```python
from build123d import *

# Parameters (mm, degrees)
SKETCH1_R      = 26.5
SKETCH1_R_2    = 5
EXTRUDE1_DEPTH = 60
SKETCH3_R      = 2
EXTRUDE2_DEPTH = 10
EXTRUDE3_START = -41
EXTRUDE3_DEPTH = 41
EXTRUDE4_DEPTH = 19
FILLET1_R      = 1


with BuildPart() as part:
    # Sketch1 → Extrude1 (new body)
    with BuildSketch(Plane(origin=(0, 0, 0), x_dir=(0, 0, -1), z_dir=(1, 0, 0))):
        Circle(SKETCH1_R)
        Circle(SKETCH1_R_2, mode=Mode.SUBTRACT)
    extrude(amount=EXTRUDE1_DEPTH)

    # Sketch2 → Cut-Revolve1 (revolve, cut)
    with BuildSketch(Plane.XY):
        Polygon((60, 16), (60, 26.5), (41, 26.5), (41, 12), (48, 12), (48, 19), (51, 19), (51, 17.5), (57, 17.5), (57, 16), align=None)
    revolve(axis=Axis((0, 0, 0), (1, 0, 0)), mode=Mode.SUBTRACT)

    # Sketch3 → Extrude2 (cut)
    with BuildSketch(Plane(origin=(60, 0, 0), x_dir=(0, 0, -1), z_dir=(1, 0, 0))):
        with Locations((0, 12.5)):
            Circle(SKETCH3_R)
        with Locations((12.5, 0)):
            Circle(SKETCH3_R)
        with Locations((0, -12.5)):
            Circle(SKETCH3_R)
        with Locations((-12.5, 0)):
            Circle(SKETCH3_R)
    extrude(amount=-EXTRUDE2_DEPTH, mode=Mode.SUBTRACT)

    # Sketch4 → Extrude3 (cut)
    with BuildSketch(Plane.ZY.offset(EXTRUDE3_START)):
        with BuildLine():
            Line((0, 14.5), (1.048050077, 26.479267192))
            ThreePointArc((1.048050077, 26.479267192), (0, 26.5), (-1.048050077, 26.479267192))
            Line((-1.048050077, 26.479267192), (0, 14.5))
        make_face()
        with BuildLine():
            Line((11.377526787, 23.933279846), (6.738485995, 12.839112372))
            Line((6.738485995, 12.839112372), (13.233531299, 22.959173534))
            ThreePointArc((13.233531299, 22.959173534), (12.315164059, 23.46458468), (11.377526787, 23.933279846))
        make_face()
        with BuildLine():
            Line((-6.738485995, 12.839112372), (-11.377526787, 23.933279846))
            ThreePointArc((-11.377526787, 23.933279846), (-12.315164059, 23.46458468), (-13.233531299, 22.959173534))
            Line((-13.233531299, 22.959173534), (-6.738485995, 12.839112372))
        make_face()
        with BuildLine():
            Line((21.196649379, 15.904466515), (11.933266055, 8.236938828))
            Line((11.933266055, 8.236938828), (22.387369981, 14.179409907))
            ThreePointArc((22.387369981, 14.179409907), (21.809072446, 15.053715788), (21.196649379, 15.904466515))
        make_face()
        with BuildLine():
            Line((-11.933266055, 8.236938828), (-21.196649379, 15.904466515))
            ThreePointArc((-21.196649379, 15.904466515), (-21.809072446, 15.053715788), (-22.387369981, 14.179409907))
            Line((-22.387369981, 14.179409907), (-11.933266055, 8.236938828))
        make_face()
        with BuildLine():
            Line((26.159875044, 4.232131575), (14.394278674, 1.747781864))
            Line((14.394278674, 1.747781864), (26.412531998, 2.151314351))
            ThreePointArc((26.412531998, 2.151314351), (26.306785164, 3.194222027), (26.159875044, 4.232131575))
        make_face()
        with BuildLine():
            Line((-14.394278674, 1.747781864), (-26.159875044, 4.232131575))
            ThreePointArc((-26.159875044, 4.232131575), (-26.306785164, 3.194222027), (-26.412531998, 2.151314351))
            Line((-26.412531998, 2.151314351), (-14.394278674, 1.747781864))
        make_face()
        with BuildLine():
            Line((25.130188598, -8.409733707), (13.557735519, -5.141770862))
            Line((13.557735519, -5.141770862), (24.38690124, -10.369621396))
            ThreePointArc((24.38690124, -10.369621396), (24.777930431, -9.397029507), (25.130188598, -8.409733707))
        make_face()
        with BuildLine():
            Line((-13.557735519, -5.141770862), (-25.130188598, -8.409733707))
            ThreePointArc((-25.130188598, -8.409733707), (-24.777930431, -9.397029507), (-24.38690124, -10.369621396))
            Line((-24.38690124, -10.369621396), (-13.557735519, -5.141770862))
        make_face()
        with BuildLine():
            Line((18.343478796, -19.125030344), (9.615278544, -10.853405848))
            Line((9.615278544, -10.853405848), (16.774525302, -20.51500185))
            ThreePointArc((16.774525302, -20.51500185), (17.572750443, -19.835534827), (18.343478796, -19.125030344))
        make_face()
        with BuildLine():
            Line((-9.615278544, -10.853405848), (-18.343478796, -19.125030344))
            ThreePointArc((-18.343478796, -19.125030344), (-17.572750443, -19.835534827), (-16.774525302, -20.51500185))
            Line((-16.774525302, -20.51500185), (-9.615278544, -10.853405848))
        make_face()
        with BuildLine():
            Line((7.354499064, -25.459013011), (3.470077132, -14.078656353))
            Line((3.470077132, -14.078656353), (5.319307772, -25.960642612))
            ThreePointArc((5.319307772, -25.960642612), (6.341865104, -25.729958162), (7.354499064, -25.459013011))
        make_face()
        with BuildLine():
            Line((-3.470077132, -14.078656353), (-7.354499064, -25.459013011))
            ThreePointArc((-7.354499064, -25.459013011), (-6.341865104, -25.729958162), (-5.319307772, -25.960642612))
            Line((-5.319307772, -25.960642612), (-3.470077132, -14.078656353))
        make_face()
    extrude(amount=EXTRUDE3_DEPTH, mode=Mode.SUBTRACT)

    # Sketch5 → Extrude4 (cut)
    with BuildSketch(Plane(origin=(60, 0, 0), x_dir=(0, 0, -1), z_dir=(1, 0, 0))):
        with BuildLine():
            Line((-5, 9.346657156), (-5, 15.198684154))
            ThreePointArc((-5, 15.198684154), (-11.313708499, 11.313708499), (-15.198684154, 5))
            Line((-15.198684154, 5), (-9.346657156, 5))
            ThreePointArc((-9.346657156, 5), (-7.495331881, 7.495331881), (-5, 9.346657156))
        make_face()
        with BuildLine():
            Line((-5, 15.198684154), (-5, 18.33030278))
            ThreePointArc((-5, 18.33030278), (-13.435028843, 13.435028843), (-18.33030278, 5))
            Line((-18.33030278, 5), (-15.198684154, 5))
            ThreePointArc((-15.198684154, 5), (-11.313708499, 11.313708499), (-5, 15.198684154))
        make_face()
        with BuildLine():
            ThreePointArc((15.198684154, 5), (11.313708499, 11.313708499), (5, 15.198684154))
            Line((5, 15.198684154), (5, 9.346657156))
            ThreePointArc((5, 9.346657156), (7.495331881, 7.495331881), (9.346657156, 5))
            Line((9.346657156, 5), (15.198684154, 5))
        make_face()
        with BuildLine():
            ThreePointArc((18.33030278, 5), (13.435028843, 13.435028843), (5, 18.33030278))
            Line((5, 18.33030278), (5, 15.198684154))
            ThreePointArc((5, 15.198684154), (11.313708499, 11.313708499), (15.198684154, 5))
            Line((15.198684154, 5), (18.33030278, 5))
        make_face()
        with BuildLine():
            ThreePointArc((5, -15.198684154), (11.313708499, -11.313708499), (15.198684154, -5))
            Line((15.198684154, -5), (9.346657156, -5))
            ThreePointArc((9.346657156, -5), (7.495331881, -7.495331881), (5, -9.346657156))
            Line((5, -9.346657156), (5, -15.198684154))
        make_face()
        with BuildLine():
            ThreePointArc((5, -18.33030278), (13.435028843, -13.435028843), (18.33030278, -5))
            Line((18.33030278, -5), (15.198684154, -5))
            ThreePointArc((15.198684154, -5), (11.313708499, -11.313708499), (5, -15.198684154))
            Line((5, -15.198684154), (5, -18.33030278))
        make_face()
        with BuildLine():
            Line((-9.346657156, -5), (-15.198684154, -5))
            ThreePointArc((-15.198684154, -5), (-11.313708499, -11.313708499), (-5, -15.198684154))
            Line((-5, -15.198684154), (-5, -9.346657156))
            ThreePointArc((-5, -9.346657156), (-7.495331881, -7.495331881), (-9.346657156, -5))
        make_face()
        with BuildLine():
            Line((-15.198684154, -5), (-18.33030278, -5))
            ThreePointArc((-18.33030278, -5), (-13.435028843, -13.435028843), (-5, -18.33030278))
            Line((-5, -18.33030278), (-5, -15.198684154))
            ThreePointArc((-5, -15.198684154), (-11.313708499, -11.313708499), (-15.198684154, -5))
        make_face()
    extrude(amount=-EXTRUDE4_DEPTH, mode=Mode.SUBTRACT)

    # Fillet1
    fillet1_edges = [part.edges().sort_by_distance(p)[0] for p in [
        (48, 19, 0),
        (44.5, 10.908712115, 5),
        (50.5, 5, 9.346657156),
        (44.5, 5, 10.908712115),
        (50.5, 9.346657156, 5),
        (48, 0, -19),
        (44.5, 5, -10.908712115),
        (50.5, 9.346657156, -5),
        (44.5, 10.908712115, -5),
        (50.5, 5, -9.346657156),
        (48, -19, 0),
        (44.5, -10.908712115, -5),
        (50.5, -5, -9.346657156),
        (44.5, -5, -10.908712115),
        (50.5, -9.346657156, -5),
        (48, 0, 19),
        (44.5, -5, 10.908712115),
        (50.5, -9.346657156, 5),
        (44.5, -10.908712115, 5),
        (50.5, -5, 9.346657156),
    ]]
    fillet(fillet1_edges, radius=FILLET1_R)


solid = part.part
```
For this review, take the finished solid that the model builds, in its own axes (mm). A direction names the side the tool comes from. Give positions to 0.01 mm unless a question says otherwise; leave off trailing zeros. Write each loop counter-clockwise with the first axis right and the second up, starting at its lowest first coordinate (ties: lowest second). Pieces come first, ordered by that corner, then holes. Notation, with made-up numbers: M -18,67.5 L 5,67.5 A17 ccw 5,97.5 Z; hole C 81.5,16.25 d4. An arc over 180 degrees is marked long. One line per item, written item: value.
1) The part is to be moulded in two halves that separate along Z. For faces 1 (the cylindrical face through (20.213, -3.12, 26.316)), 2 (the flat face through (20.787, -20.103, -4.408)), 3 (the flat face through (57, 17, 0)), say which applies: +Z half, -Z half, draft (parallel to the pull), parting line (faces both ways), or undercut.
Results are:
face 1: +Z half
face 2: undercut
face 3: draft
2) Take a section at C-C, the plane y = -6.5. Write out the cut boundary in (x, z).
Results are:
outline: M 0,-25.69 L 41,-25.69 L 41,-18.37 L 0,-18.37 Z; M 0,-16.37 L 41,-16.37 L 41,-8.37 L 60,-8.37 L 60,8.37 L 41,8.37 L 41,16.37 L 0,16.37 Z; M 0,18.37 L 41,18.37 L 41,25.69 L 0,25.69 Z
3) Take a section at B-B, the plane z = -20. Write out the cut boundary in (x, y), then the cut area to 3 significant figures.
Results are:
outline: M 0,-17.39 L 41,-17.39 L 41,-8.25 L 0,-8.25 Z; M 0,-6.96 L 41,-6.96 L 41,1.94 L 0,1.94 Z; M 0,2.93 L 41,2.93 L 41,12.82 L 0,12.82 Z; M 0,14.91 L 41,14.91 L 41,17.39 L 0,17.39 Z
area: 1,250 mm²
4) For P1, Ø2.5, axis at x = 53.5, y = 12.5, coming from the +Z side; P2, Ø2, axis at y = -1.5, z = 17.5, coming from the +X side; P3, Ø4, axis at y = -13.5, z = 18, coming from the +X side, all flat-tipped, find the tip position at first contact; note any pin that passes through.
Results are:
P1: stops at z = 5
P2: stops at x = 57
P3: stops at x = 41
5) For line 1 (Y direction, x = 52, z = 0); line 2 (X direction, y = 3.5, z = 12.5); line 3 (Z direction, x = 33.5, y = -21.5), list the stretches that pass through material, from the lowest coordinate up. Write a range as from..to.
Results are:
line 1: y = -17.5..-14.5, -10.5..-5, 5..10.5, 14.5..17.5
line 2: x = 0..41, 48..60
line 3: z = -15.49..-6, -4.63..4.63, 6..15.49
6) For faces 4 (the cylindrical face through (50.63, 7.52, -7.47)), 5 (the cylindrical face through (45, -12, 0)), 6 (the cylindrical face through (59, 16, 0)), list the 3-axis set-ups (+Z, -Z, +X, -X, +Y, -Y) from which the entire face can be reached by the end or side of a thin tool; tool diameter is ignored.
Results are:
face 4: -Z, +X, +Y
face 5: -Y
face 6: +X, +Y
